Check sheet for the drawn part. Datum: minimum x, y, z corner. Units: mm. Give positions to 0.01 mm unless a question says otherwise; leave off trailing zeros. Loops run counter-clockwise (first coordinate to the right, second up) from the corner with the lowest first, then second, coordinate; pieces in that order, holes last. Notation, with made-up numbers: (48.5, -26.75) - (58.5, -26.75) arc R12 ccw to (58.5, -15.75) - close; hole circle Ø7 at (62, 25). An arc over 180 degrees is marked (long way). One line per item, written item: value. Start each with the question number.
1. Sectioned sample at B-B (x = 6). Record the cut outline in (y, z).
2. Sectioned sample at D-D (x = 14.75). Count the separate pieces of the cut face and the enclosed holes in it, plus the area to 3 significant figures.
3. Sectioned sample at A-A (y = 4.5). Record the cut outline in (x, z), plus the area to 3 significant figures.
4. Mould release check, pull along Z, two halves, no side actions. Record for the marked faces 1, 2 and 3: pulls with the +Z half, pulls with the -Z half, needs draft (parallel to the pull), parting line crosses it, or undercut.
5. Gauge pin test, flat ends, axial feed: pin 1 (3.5 mm diameter, centred on x = 6, z = 33, fed in from +Y); pin 2 (6 mm diameter, centred on y = 11.5, z = 21.5, fed in from +X). Record the tip position at first contact, or that the pin passes through.
6. Scan lines: L1, parallel to Z at x = 10.25, y = 4.5; L2, parallel to Y at x = 6, z = 5; L3, parallel to X at y = 8.5, z = 15. Record each from-to range of solid material in increasing order. Write a range as [from, to].
7. Sectioned sample at C-C (z = 37). Record the cut outline in (x, y).
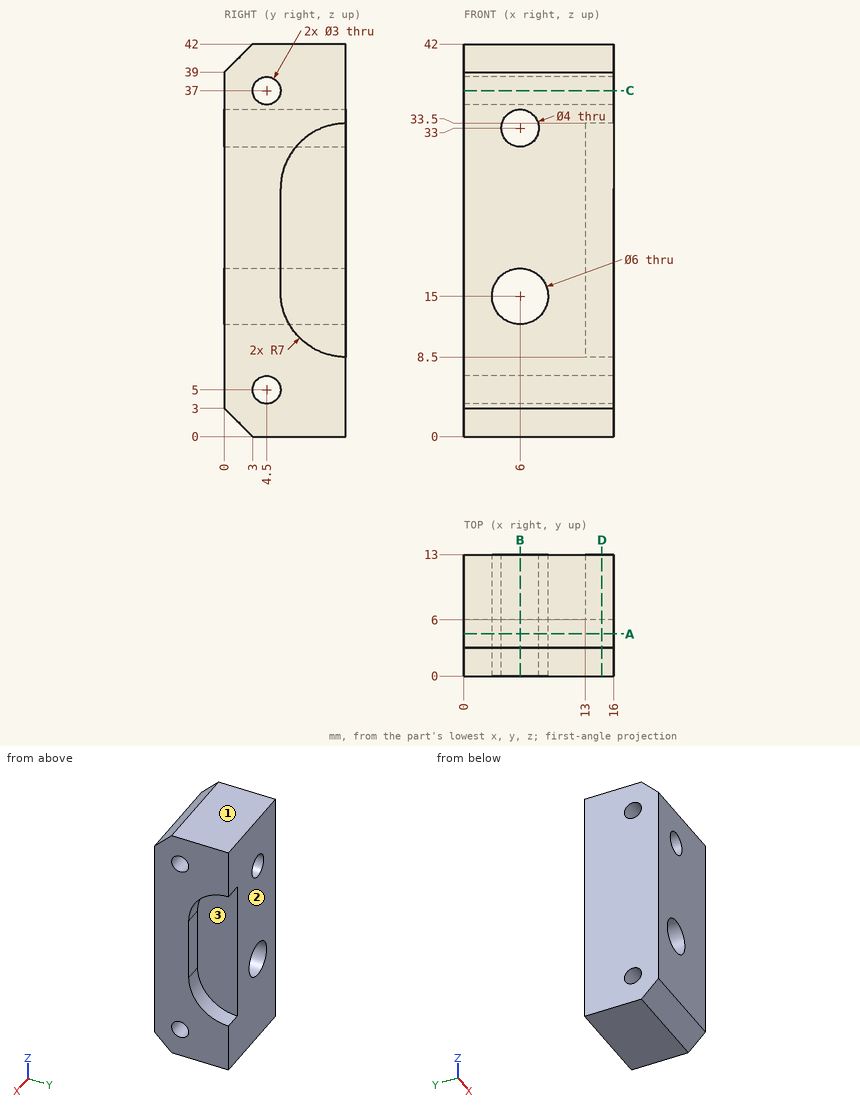
Results are:
1. outline: (0, 3) - (3, 0) - (13, 0) - (13, 12) - (0, 12) - close; (0, 18) - (13, 18) - (13, 31) - (0, 31) - close; (0, 35) - (13, 35) - (13, 42) - (3, 42) - (0, 39) - close; hole circle Ø3 at (4.5, 5); hole circle Ø3 at (4.5, 37)
2. separate pieces: 1
2. enclosed holes: 2
2. area: 369 mm^2
3. outline: (0, 0) - (16, 0) - (16, 3.5) - (0, 3.5) - close; (0, 6.5) - (16, 6.5) - (16, 35.5) - (0, 35.5) - close; (0, 38.5) - (16, 38.5) - (16, 42) - (0, 42) - close; hole circle Ø6 at (6, 15); hole circle Ø4 at (6, 33)
3. area: 535 mm^2
4. face 1: pulls with the +Z half
4. face 2: needs draft
4. face 3: undercut
5. pin 1: passes through
5. pin 2: stops at x = 13
6. L1: z = [0, 3.5], [6.5, 35.5], [38.5, 42]
6. L2: y = [0, 3], [6, 13]
6. L3: x = [0, 3], [9, 13]
7. outline: (0, 0) - (16, 0) - (16, 3) - (0, 3) - close; (0, 6) - (16, 6) - (16, 13) - (0, 13) - close
